from build123d import *

# Parameters (mm, degrees)
CROQUIS1_W              = 360
CROQUIS1_H              = 35
SALIENTE_EXTRUIR1_DEPTH = 4
CROQUIS2_R              = 2
CORTAR_EXTRUIR1_DEPTH   = 5
TALADRO_ROSCADO_M31_D   = 2.5
CHAFL_N1_SIZE           = 8
REDONDEO2_R             = 4


with BuildPart() as part:
    # Croquis1 → Saliente-Extruir1 (new body)
    with BuildSketch(Plane.XY):
        Rectangle(CROQUIS1_W, CROQUIS1_H)
    extrude(amount=SALIENTE_EXTRUIR1_DEPTH)

    # Croquis2 → Cortar-Extruir1 (cut)
    with BuildSketch(Plane.XY.offset(4)):
        with Locations((0, 14)):
            Circle(CROQUIS2_R)
        with Locations((0, -14)):
            Circle(CROQUIS2_R)
        with Locations((161, 14)):
            Circle(CROQUIS2_R)
        with Locations((161, -14)):
            Circle(CROQUIS2_R)
        with Locations((-161, 14)):
            Circle(CROQUIS2_R)
        with Locations((-161, -14)):
            Circle(CROQUIS2_R)
    extrude(amount=-CORTAR_EXTRUIR1_DEPTH, mode=Mode.SUBTRACT)

    # Taladro roscado M31 (through all)
    with Locations(Plane.XY.offset(4)):
        with Locations((-170, 0), (-110, 0), (-50, 0), (50, 0), (110, 0), (170, 0)):
            Hole(TALADRO_ROSCADO_M31_D / 2)

    # Chaflán1
    chafl_n1_edges = [part.edges().sort_by_distance(p)[0] for p in [
        (180, -17.5, 2),
        (-180, -17.5, 2),
        (-180, 17.5, 2),
        (180, 17.5, 2),
    ]]
    chamfer(chafl_n1_edges, length=CHAFL_N1_SIZE)

    # Redondeo2
    redondeo2_edges = [part.edges().sort_by_distance(p)[0] for p in [
        (180, 9.5, 2),
        (180, -9.5, 2),
        (-172, -17.5, 2),
        (172, -17.5, 2),
        (-172, 17.5, 2),
        (172, 17.5, 2),
        (-180, 9.5, 2),
        (-180, -9.5, 2),
    ]]
    fillet(redondeo2_edges, radius=REDONDEO2_R)


solid = part.part
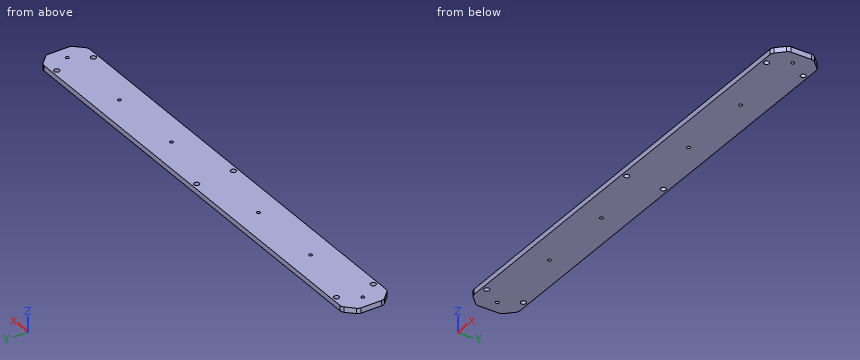
The listing builds one solid part. Answer for the finished solid, in the listing's coordinates (mm). Round coordinates to 2 decimals unless told otherwise and drop trailing zeros. Write each question's results on one line, items separated by ' | '. Start each with the question number.
1) This flat-tipped pin is pushed along its axis until it touches: pin 1 (2 mm diameter, centred on x = 170, y = 0, fed in from -Z). Where does it stop, or does it pass through?
2) Straight lines are drawn through the part: probe 1 along Y at (x, z) = (0, 2.1); probe 2 along Y at (x, z) = (-50, 0.9); probe 3 along Y at (x, z) = (49, 3.45). For each, find the intervals that lie inside material, in ascending order.
3) Find section A-A on z = 3.05. Count the separate pieces of the cut face and the enclosed holes in it, plus the area to 3 significant figures.
Final values:
1) pin 1: through
2) probe 1: -17.5 to -16, -12 to 12, 16 to 17.5 | probe 2: -17.5 to -1.25, 1.25 to 17.5 | probe 3: -17.5 to -0.75, 0.75 to 17.5
3) separate pieces: 1 | enclosed holes: 12 | area: 12,400 mm²
